```python
from build123d import *

# Parameters (mm, degrees)
F0_W     = 25.4
F0_H     = 25.4
F1_DEPTH = 1.5875
F2_W     = 12.7
F2_H     = 25.4
F3_DEPTH = 3.175
F5_DEPTH = 3.175


with BuildPart() as f1:
    # F0 (on Front) → F1 (new body, symmetric)
    with BuildSketch(Plane.XZ):
        with Locations((-0.326153, 40.037792)):
            Rectangle(F0_W, F0_H)
    extrude(amount=F1_DEPTH, both=True)

    # F2 (on face) → F3 (join)
    with BuildSketch(Plane.XZ.offset(1.5875)):
        with Locations((-6.676153, 14.637792)):
            Rectangle(F2_W, F2_H)
    extrude(amount=-F3_DEPTH)

    # F4 (on face) → F5 (join)
    with BuildSketch(Plane.XZ.offset(1.5875)):
        with BuildLine():
            Line((12.373847, 1.937792), (-13.026153, 1.937792))
            ThreePointArc((-13.026153, 1.937792), (-0.326153, -10.762208), (12.373847, 1.937792))
        make_face()
    extrude(amount=-F5_DEPTH)


solid = f1.part
```
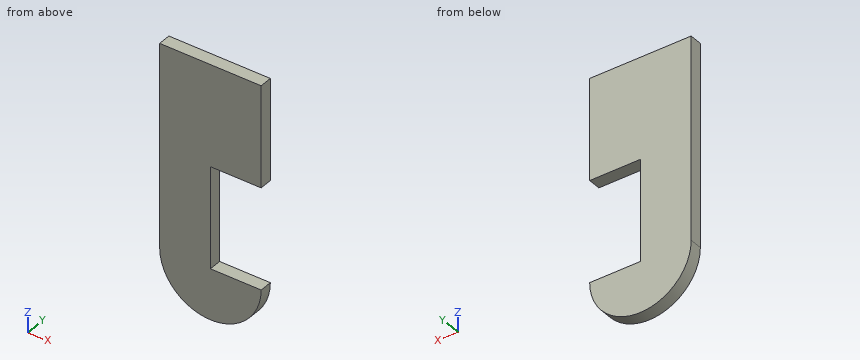
Source: CAD feature listing. Evaluate the final solid. Frame: model axes, mm. Round coordinates to 2 decimals unless told otherwise and drop trailing zeros. Loops run counter-clockwise (first coordinate to the right, second up) from the corner with the lowest first, then second, coordinate; pieces in that order, holes last. Notation, with made-up numbers: M 67.25,55.25 L 74.25,55.25 A30 ccw 74.25,77.25 Z; hole C 26.5,-29 d9. An arc over 180 degrees is marked long. Put each result on its own line as item: value.
(1) Section A-A, the plane x = 6.5. Return loops of the section in (y, z).
Solutions:
outline: M -1.59,-8.77 L 1.59,-8.77 L 1.59,1.94 L -1.59,1.94 Z; M -1.59,27.34 L 1.59,27.34 L 1.59,52.74 L -1.59,52.74 Z
(2) Section D-D, the plane x = 10. Return loops of the section in (y, z).
Solutions:
outline: M -1.59,-5.46 L 1.59,-5.46 L 1.59,1.94 L -1.59,1.94 Z; M -1.59,27.34 L 1.59,27.34 L 1.59,52.74 L -1.59,52.74 Z
(3) First-contact query: pin 1 (1 mm diameter, centred on x = 5.5, y = 0.5, fed in from -Z); pin 2 (1 mm diameter, centred on y = 0, z = 18.5, fed in from +X). Flat tips, straight axial feed; report the tip coordinate or a pass-through.
Solutions:
pin 1: z = -9.59
pin 2: x = -0.33
(4) Section C-C, the plane z = 8. Return loops of the section in (x, y), and give its area (3 significant figures).
Solutions:
outline: M -13.03,-1.59 L -0.33,-1.59 L -0.33,1.59 L -13.03,1.59 Z
area: 40.3 mm²
(5) Ray query, line 1 (Z direction, x = 6, y = 1); line 2 (X direction, y = 1.1, z = 18); line 3 (Z direction, x = 1.75, y = 0.85). Return the intervals inside material, ascending. Write a range as [from, to].
Solutions:
line 1: [-9.07, 1.94], [27.34, 52.74]
line 2: [-13.03, -0.33]
line 3: [-10.59, 1.94], [27.34, 52.74]
(6) Section B-B, the plane y = -1.1. Return loops of the section in (x, z), and give its area (3 significant figures).
Solutions:
outline: M -13.03,1.94 A12.7 ccw 12.37,1.94 L -0.33,1.94 L -0.33,27.34 L 12.37,27.34 L 12.37,52.74 L -13.03,52.74 Z
area: 1,220 mm²
